Build history of the part. All positions in model axes, mm. A direction names the side the tool comes from. Give positions to 0.01 mm unless a question says otherwise; leave off trailing zeros. Order: outer loops, then holes, each group sorted by start corner. A loop starts at its lowest first (then second) coordinate and runs counter-clockwise, first axis right, second up. Notation, with made-up numbers: (-9, 65) - (12, 65) arc R35 ccw to (12, 99) - close; hole circle Ø5 at (-8.75, -24). An arc over 180 degrees is marked (long way). Use a Markdown table: item, result.
from build123d import *

# Parameters (mm, degrees)
SKETCH_W        = 53
SKETCH_H        = 26
PAD_DEPTH       = 16
FILLET_R        = 3
SKETCH001_W     = 3.5
SKETCH001_H     = 2
POCKET_DEPTH    = 3
SKETCH002_W     = 26
SKETCH002_H     = 0.5
POCKET001_DEPTH = 0.3
SKETCH003_W     = 53
SKETCH003_H     = 0.5
POCKET002_DEPTH = 0.1
SKETCH004_W     = 26
SKETCH004_H     = 0.5
POCKET003_DEPTH = 0.1
SKETCH005_W     = 53
SKETCH005_H     = 0.5
POCKET004_DEPTH = 0.1
SKETCH006_W     = 3.1
SKETCH006_H     = 1
PAD001_DEPTH    = 3
POCKET005_DEPTH = 1


with BuildPart() as part:
    # Sketch → Pad (new body)
    with BuildSketch(Plane.XY):
        Rectangle(SKETCH_W, SKETCH_H)
    extrude(amount=PAD_DEPTH)

    # Fillet
    fillet_edges = [part.edges().sort_by_distance(p)[0] for p in [
        (0, -13, 16),
        (0, -13, 0),
        (0, 13, 16),
        (0, 13, 0),
    ]]
    fillet(fillet_edges, radius=FILLET_R)

    # Sketch001 (on Face2 of Fillet) → Pocket (cut)
    with BuildSketch(Plane(origin=(-26.5, 0, 0), x_dir=(0, -1, 0), z_dir=(-1, 0, 0))):
        with Locations((-2.45, 2)):
            Rectangle(SKETCH001_W, SKETCH001_H)
        with Locations((2.45, 2)):
            Rectangle(SKETCH001_W, SKETCH001_H)
    extrude(amount=-POCKET_DEPTH, mode=Mode.SUBTRACT)

    # Sketch002 (on Face2 of Pocket) → Pocket001 (cut)
    with BuildSketch(Plane(origin=(-26.5, 0, 0), x_dir=(0, -1, 0), z_dir=(-1, 0, 0))):
        with Locations((0, 5.75)):
            Rectangle(SKETCH002_W, SKETCH002_H)
    extrude(amount=-POCKET001_DEPTH, mode=Mode.SUBTRACT)

    # Sketch003 (on Face1 of Pocket001) → Pocket002 (cut)
    with BuildSketch(Plane(origin=(0, 13, 0), x_dir=(-1, 0, 0), z_dir=(0, 1, 0))):
        with Locations((0, 5.75)):
            Rectangle(SKETCH003_W, SKETCH003_H)
    extrude(amount=-POCKET002_DEPTH, mode=Mode.SUBTRACT)

    # Sketch004 (on Face3 of Pocket002) → Pocket003 (cut)
    with BuildSketch(Plane.YZ.offset(26.5)):
        with Locations((0, 5.75)):
            Rectangle(SKETCH004_W, SKETCH004_H)
    extrude(amount=-POCKET003_DEPTH, mode=Mode.SUBTRACT)

    # Sketch005 (on Face10 of Pocket003) → Pocket004 (cut)
    with BuildSketch(Plane.XZ.offset(13)):
        with Locations((0, 5.75)):
            Rectangle(SKETCH005_W, SKETCH005_H)
    extrude(amount=-POCKET004_DEPTH, mode=Mode.SUBTRACT)

    # Sketch006 (on Face7 of Pocket004) → Pad001 (join)
    with BuildSketch(Plane(origin=(-26.5, 0, 0), x_dir=(0, -1, 0), z_dir=(-1, 0, 0))):
        with Locations((-2.45, 1.9)):
            Rectangle(SKETCH006_W, SKETCH006_H)
        with Locations((2.45, 1.9)):
            Rectangle(SKETCH006_W, SKETCH006_H)
    extrude(amount=-PAD001_DEPTH)

    # Sketch007 (on Face45 of Pad001) → Pocket005 (cut)
    with BuildSketch(Plane.YZ.offset(26.5)):
        with BuildLine():
            ThreePointArc((-3.7, 12.5), (-5.45, 10.75), (-3.7, 9))
            Line((-3.7, 9), (3.7, 9))
            ThreePointArc((3.7, 9), (5.45, 10.75), (3.7, 12.5))
            Line((-3.7, 12.5), (3.7, 12.5))
        make_face()
    extrude(amount=-POCKET005_DEPTH, mode=Mode.SUBTRACT)


solid = part.part
1) Pin check, flat tip, straight feed: P1, Ø1.6, axis at x = -25.5, z = 1.5, coming from the +Y side. Stop position of the tip, or through.
Computed:
| item | result |
|---|---|
| P1 | stops at y = 12.92 |
2) Slice it at A-A (x = 12). Write the cut outline in (y, z), and give its area (3 significant figures).
Computed:
| item | result |
|---|---|
| outline | (-13, 3) arc R3 ccw to (-10, 0) - (10, 0) arc R3 ccw to (13, 3) - (13, 5.5) - (12.9, 5.5) - (12.9, 6) - (13, 6) - (13, 13) arc R3 ccw to (10, 16) - (-10, 16) arc R3 ccw to (-13, 13) - (-13, 6) - (-12.9, 6) - (-12.9, 5.5) - (-13, 5.5) - close |
| area | 408 mm² |
3) Two-plate mould, pull along Y, no slides. Class faces 4 (the flat face through (-25, 4, 2)), 5 (the flat face through (-26.5, 0, 11)), 6 (the flat face through (0, -13, 4)): +Y half, -Y half, draft (parallel to the pull), parting line (faces both ways), or undercut.
Computed:
| item | result |
|---|---|
| face 4 | undercut |
| face 5 | draft |
| face 6 | -Y half |
4) Wall check: line 1 (Y direction, x = 23, z = 2.75); line 2 (Y direction, x = -11.5, z = 13.75); line 3 (Z direction, x = -2.5, y = 10.75). Give the ranges that are in metal, low to high. Write a range as from..to.
Computed:
| item | result |
|---|---|
| line 1 | y = -12.99..12.99 |
| line 2 | y = -12.9..12.9 |
| line 3 | z = 0.1..15.9 |
5) Tool access for faces 1 (the flat face through (26, 0, 12.5)), 2 (the flat face through (-25, 4.2, 2)), 3 (the flat face through (0, 13, 9)): list every direction of +Z, -Z, +X, -X, +Y, -Y with a clear straight run to the whole face (end or side of a thin tool).
Computed:
| item | result |
|---|---|
| face 1 | +X |
| face 2 | -X |
| face 3 | +Z, -Z, +X, -X, +Y |
6) Slice it at B-B (y = -11). Write the cut outline in (x, z).
Computed:
| item | result |
|---|---|
| outline | (-26.5, 0.17) - (26.5, 0.17) - (26.5, 5.5) - (26.4, 5.5) - (26.4, 6) - (26.5, 6) - (26.5, 15.83) - (-26.5, 15.83) - (-26.5, 6) - (-26.2, 6) - (-26.2, 5.5) - (-26.5, 5.5) - close |
